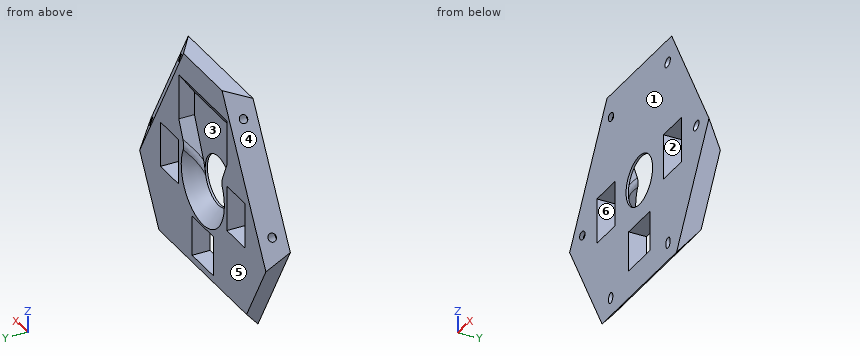
```python
from build123d import *

# Parameters (mm, degrees)
BOSS_EXTRUDE1_DEPTH = 8
CHAMFER1_SIZE       = 10
CHAMFER1_SIZE_2     = 11.917535926
SKETCH4_R           = 1.85
CUT_EXTRUDE1_DEPTH  = 101.029376687
SKETCH5_R           = 11.15
CUT_EXTRUDE3_DEPTH  = 79.744901298
SKETCH6_R           = 1.85
CUT_EXTRUDE4_DEPTH  = 101.029376687
SKETCH7_R           = 1.85
CUT_EXTRUDE5_DEPTH  = 97.338690096
SKETCH8_W           = 15.4
SKETCH8_H           = 20.4
CUT_EXTRUDE6_DEPTH  = 79.744901298
SKETCH9_W           = 40.4
SKETCH9_H           = 10.4
CUT_EXTRUDE7_DEPTH  = 7
CUT_EXTRUDE8_DEPTH  = 7
CHAMFER2_SIZE       = 7
CHAMFER3_SIZE       = 10
CHAMFER3_SIZE_2     = 7.002075382
FILLET1_R           = 3
SKETCH11_W          = 18
SKETCH11_H          = 18
CUT_EXTRUDE9_DEPTH  = 79.744901364


with BuildPart() as part:
    # Sketch1 → Boss-Extrude1 (new body)
    with BuildSketch(Plane(origin=(0, 0, 0), x_dir=(1, 0, 0), z_dir=(0, 1, 0))):
        Polygon((-60, 0), (-30, -51.961524227), (30, -51.961524227), (60, 0), (30, 51.961524227), (-30, 51.961524227), align=None)
    extrude(amount=BOSS_EXTRUDE1_DEPTH)

    # Chamfer1
    # the kernel refuses this chamfer: 11.917535926, 10 mm, written as the material it takes off along each edge
    with BuildSketch(Plane(origin=(60.716329832, 8, -51.961524227), x_dir=(0, -0.9993728857116146, -0.0354095369136628), z_dir=(-1, 0, 0)), Plane(origin=(-75.358164916, 8, -26.601121946), x_dir=(-0.030665558503474466, -0.9993728857116146, 0.017704768456831187), z_dir=(0.4999999999999998, 0, 0.8660254037844388)), Plane(origin=(14.641835084, 8, 78.562646173), x_dir=(0.03066555850347504, -0.9993728857116146, 0.017704768456831523), z_dir=(0.4999999999999999, 0, -0.8660254037844388))) as chamfer1_piece_1:
        Polygon((CHAMFER1_SIZE * 0.999372885712, CHAMFER1_SIZE * 0.0354095369137), (-CHAMFER1_SIZE_2 * 0.0354095369135, CHAMFER1_SIZE_2 * 0.999372885707), (0, 0), align=None)
    extrude(amount=121.432659665, mode=Mode.SUBTRACT)

    # Sketch4 → Cut-Extrude1 (cut, through all)
    with BuildSketch(Plane(origin=(17.740047471, 24.412407781, 10.242221183), x_dir=(0.8301060005968394, -0.4979011414928883, -0.251034820439713), z_dir=(0.5566703992264198, 0.7660444431189777, 0.3213938048432698))):
        with Locations(Location((39.858257334, -1.394557769, 0), (0, 0, 164.627134315))):
            Circle(SKETCH4_R)
        with Locations(Location((9.338033447, -38.774045448, 0), (0, 0, 164.627134315))):
            Circle(SKETCH4_R)
    extrude(amount=-CUT_EXTRUDE1_DEPTH, mode=Mode.SUBTRACT)

    # Sketch5 → Cut-Extrude3 (cut, through all)
    with BuildSketch(Plane(origin=(0, 0, 0), x_dir=(1, 0, 0), z_dir=(0, 1, 0))):
        with Locations(Location((0, 0, 0), (0, 0, 270))):
            Circle(SKETCH5_R)
    extrude(amount=CUT_EXTRUDE3_DEPTH, mode=Mode.SUBTRACT)

    # Sketch6 → Cut-Extrude4 (cut, through all)
    with BuildSketch(Plane(origin=(-17.740047471, 24.412407781, 10.242221183), x_dir=(0.8307334510088673, 0.5133226132381532, 0.21536440772154375), z_dir=(-0.5566703992264165, 0.7660444431189809, 0.3213938048432678))):
        with Locations(Location((-39.882343662, 0.155348314, 0), (0, 0, 193.145847187))):
            Circle(SKETCH6_R)
        with Locations(Location((-10.837701827, -38.381892712, 0), (0, 0, 193.145847187))):
            Circle(SKETCH6_R)
    extrude(amount=-CUT_EXTRUDE4_DEPTH, mode=Mode.SUBTRACT)

    # Sketch7 → Cut-Extrude5 (cut, through all)
    with BuildSketch(Plane(origin=(0, 24.412407781, -20.484442365), x_dir=(1, 0, 0), z_dir=(0, 0.7660444431189811, -0.6427876096865357))):
        with Locations(Location((-24.128355545, 31.756069148, 0), (0, 0, 270))):
            Circle(SKETCH7_R)
        with Locations(Location((24.128355545, 31.756069148, 0), (0, 0, 270))):
            Circle(SKETCH7_R)
    extrude(amount=-CUT_EXTRUDE5_DEPTH, mode=Mode.SUBTRACT)

    # Sketch8 → Cut-Extrude6 (cut, through all)
    with BuildSketch(Plane(origin=(0, 8, 0), x_dir=(1, 0, 0), z_dir=(0, 1, 0))):
        with Locations((-28, 0)):
            Rectangle(SKETCH8_W, SKETCH8_H)
        with Locations((28, 0)):
            Rectangle(SKETCH8_W, SKETCH8_H)
    extrude(amount=-CUT_EXTRUDE6_DEPTH, mode=Mode.SUBTRACT)

    # Sketch9 → Cut-Extrude7 (cut)
    with BuildSketch(Plane(origin=(0, 8, 0), x_dir=(1, 0, 0), z_dir=(0, 1, 0))):
        with Locations((0, -25)):
            Rectangle(SKETCH9_W, SKETCH9_H)
    extrude(amount=-CUT_EXTRUDE7_DEPTH, mode=Mode.SUBTRACT)

    # Sketch10 → Cut-Extrude8 (cut)
    with BuildSketch(Plane(origin=(0, 8, 0), x_dir=(1, 0, 0), z_dir=(0, 1, 0))):
        Polygon((-20.2, -19.8), (-11.15, 0), (11.15, 0), (20.2, -19.8), align=None)
    extrude(amount=-CUT_EXTRUDE8_DEPTH, mode=Mode.SUBTRACT)

    # Chamfer2
    chamfer2_edges = [part.edges().sort_by_distance(p)[0] for p in [
        (0, 8, -11.15),
    ]]
    chamfer(chamfer2_edges, length=CHAMFER2_SIZE)

    # Chamfer3
    # the kernel refuses this chamfer: 10, 7.002075382 mm, written as the material it takes off along each edge
    with BuildSketch(Plane(origin=(20.2, 8, 30.2), x_dir=(0, 0.02220967419845712, 0.9997533347641299), z_dir=(-1, 0, 0))) as chamfer3_piece_1_section:
        Polygon((CHAMFER3_SIZE * 0.999753334764, -CHAMFER3_SIZE * 0.0222096741985), (-CHAMFER3_SIZE_2 * 0.0222096741988, -CHAMFER3_SIZE_2 * 0.999753334778), (0, 0), align=None)
    chamfer3_piece_1 = extrude(amount=40.4, mode=Mode.PRIVATE)
    chamfer3_piece_1 = split(chamfer3_piece_1, bisect_by=Plane(origin=(0, 1, 33.539189969), z_dir=(0, 1, 0)), keep=Keep.TOP, mode=Mode.PRIVATE)
    add(chamfer3_piece_1, mode=Mode.SUBTRACT)

    # Fillet1
    fillet1_edges = [part.edges().sort_by_distance(p)[0] for p in [
        (-13.4116744, 4.145370972, 4.948193714),
        (13.4116744, 4.145370972, 4.948193714),
    ]]
    fillet(fillet1_edges, radius=FILLET1_R)

    # Sketch11 → Cut-Extrude9 (cut, through all)
    with BuildSketch(Plane(origin=(0, 8, 0), x_dir=(1, 0, 0), z_dir=(0, 1, 0))):
        with Locations((0, 28)):
            Rectangle(SKETCH11_W, SKETCH11_H)
    extrude(amount=-CUT_EXTRUDE9_DEPTH, mode=Mode.SUBTRACT)


solid = part.part
```
Can you work these out from the model? Positions are in its coordinate system, mm. Face numbers are marked on the shaded views. A direction names the side the tool comes from. Give positions to 0.01 mm unless a question says otherwise; leave off trailing zeros. Write each loop counter-clockwise with the first axis right and the second up, starting at its lowest first coordinate (ties: lowest second). Pieces come first, ordered by that corner, then holes. Notation, with made-up numbers: (44.25, 64.5) - (98.25, 64.5) arc R34 ccw to (98.25, 103.5) - close; hole circle Ø7 at (-22.5, -18). An arc over 180 degrees is marked (long way). Write item = value, one per line. Start each with the question number.
1. Imagine slicing it at A-A (x = 0). Please give me the cut outline in (y, z), and give its area (3 significant figures).
2. Imagine slicing it at D-D (z = -6.5). Count the separate pieces of the cut face and the enclosed holes in it, and give its area (3 significant figures).
3. Please list where these lines run through material, in increasing order: line 1 (X direction, y = 0.6, z = 0); line 2 (X direction, y = 1.5, z = -10); line 3 (Z direction, x = 0, y = 0.45).
4. Imagine slicing it at B-B (z = -33). Please give me the cut outline in (x, y).
5. On a 3-axis mill with a long thin cutter (end or side, diameter ignored), from which of +Z, -Z, +X, -X, +Y, -Y can I reach the whole of each face in a straight line? I mean the marked faces 1, 2 and 3. Say none if no direction works.
6. Thinking about a two-plate mould opening in Z: for the marked faces 4, 5 and 6, which applies, released by +Z, released by -Z, zero draft, split by the parting line, or undercut?
7. Imagine slicing it at C-C (z = 35). Please give me the cut outline in (x, y).
8. For pin 1 (2.5 mm diameter, centred on y = 2, z = -27, fed in from -X); pin 2 (10 mm diameter, centred on x = -7.5, z = 13, fed in from +Y); pin 3 (2.5 mm diameter, centred on x = 29.5, y = 3, fed in from -Z); pin 4 (12 mm diameter, centred on x = 28, z = -4, fed in from -Y), each with a flat end and sliding along its axis, tell me the tip position at first contact or that it passes through.
Worked answers:
q1.outline = (0, -49.58) - (8, -40.04) - (8, -37) - (0, -37) - close; (0, -19) - (8, -19) - (8, -18.15) - (1, -11.15) - (0, -11.15) - close; (0, 11.15) - (1, 11.15) - (1, 30.2) - (8, 40.2) - (8, 51.96) - (0, 51.96) - close
q1.area = 259 mm2
q2.separate_pieces = 4
q2.enclosed_holes = 0
q2.area = 424 mm2
q3.line_1 = -56.42 to -50.6, -46.15 to -35.7, -20.3 to -11.15, 11.15 to 20.3, 35.7 to 46.15, 50.6 to 56.42
q3.line_2 = -54.23 to -35.7, -20.3 to -5.98, 5.98 to 20.3, 35.7 to 54.23
q3.line_3 = -49.04 to -37, -19 to -11.15, 11.15 to 51.96
q4.outline = (-40.95, 0) - (-9, 0) - (-9, 8) - (-40.95, 8) - close; (9, 0) - (40.95, 0) - (40.95, 8) - (9, 8) - close
q5.face_1 = +Z, -Z, +X, -X, -Y
q5.face_2 = +Y, -Y
q5.face_3 = +Y
q6.face_4 = released by +Z
q6.face_5 = zero draft
q6.face_6 = undercut
q7.outline = (-37.04, 0) - (37.04, 0) - (26.03, 8) - (20.2, 8) - (20.2, 4.36) - (-20.2, 4.36) - (-20.2, 8) - (-26.03, 8) - close
q8.pin_1 = -45.13
q8.pin_2 = 1
q8.pin_3 = -47.49
q8.pin_4 = through
